Autodesk Inventor part; units mm, degrees
ref_plane "YZ Plane" through (0, 0, 0) normal (1, 0, 0) x (0, 1, 0)
ref_plane "XZ Plane" through (0, 0, 0) normal (0, 1, 0) x (-1, 0, 0)
ref_plane "XY Plane" through (0, 0, 0) normal (0, 0, 1) x (1, 0, 0)
sketch "Sketch1" plane through (0, 0, 0) normal (0, 1, 0) x (-1, 0, 0)
  circle A0 centre (0, 0) radius 175
  dimension "d0" = 350
extrude "Extrusion1" add sketch "Sketch1" along normal blind 10
sketch "Sketch2" plane through (0, 0, 0) normal (0, -1, 0) x (1, 0, 0)
  circle A0 centre (0, 0) radius 175
  circle A1 centre (0, 135) radius 25
  line L0 (-25, 135) -> (-25, 173.2051)
  line L1 (25, 135) -> (25, 173.2051)
  dimension "d3" = 50
  dimension "d4" = 135
extrude "Extrusion2" cut sketch "Sketch2" against normal through all contours L1 A1 L0 A0 | A1 picked at (-14.0746, 168.7936)
pattern_circular "Circular Pattern1" count 4 over 360 about axis through (0, 0, 0) along (0, 1, 0) of "Extrusion2"
properties part number "Base" material "Steel"
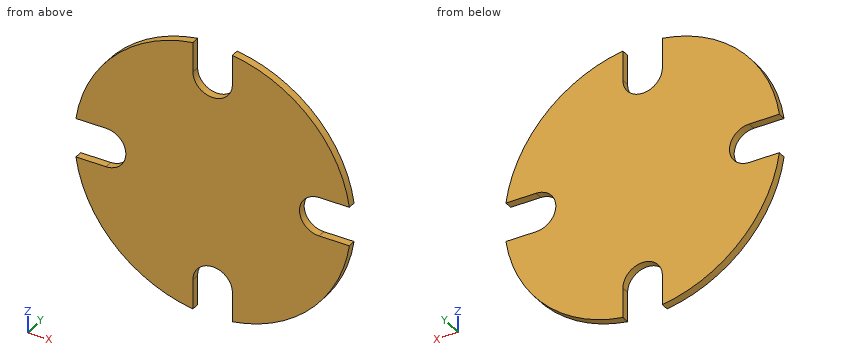
Check sheet for the modelled part. Datum: model origin and axes. Units: mm. Give positions to 0.01 mm unless a question says otherwise; leave off trailing zeros. Write each loop counter-clockwise with the first axis right and the second up, starting at its lowest first coordinate (ties: lowest second). Pieces come first, ordered by that corner, then holes.
Item 1: Gauge pin test, flat ends, axial feed: pin 1 (1.5 mm diameter, centred on y = 8, z = -119, fed in from +X); pin 2 (5 mm diameter, centred on y = 6, z = -151.5, fed in from +X); pin 3 (5 mm diameter, centred on x = 158.5, y = 5.5, fed in from +Z). Record the tip position at first contact, or that the pin passes through.
Item 2: Scan lines: L1, parallel to Z at x = 129.5, y = 5; L2, parallel to X at y = 4.25, z = -147; L3, parallel to Z at x = -117, y = 4.25. Record each from-to range of solid material in increasing order.
Item 3: Cross-section at D-D (z = 0). Enter the section's corners in (x, y), and give its area (3 significant figures).
Item 4: Cross-section at A-A (y = 2.5). Enter the section's corners in (x, z).
Item 5: Cross-section at C-C (x = 0). Enter the section's corners in (y, z), and give its area (3 significant figures).
Item 6: Cross-section at B-B (x = 152). Enter the section's corners in (y, z), and give its area (3 significant figures).
Report:
1. pin 1: stops at x = 129
1. pin 2: stops at x = 91.78
1. pin 3: stops at z = 79.3
2. L1: z = -117.71 to -24.39, 24.39 to 117.71
2. L2: x = -94.95 to -25, 25 to 94.95
2. L3: z = -130.14 to -17.35, 17.35 to 130.14
3. outline: (-110, 0) - (110, 0) - (110, 10) - (-110, 10) - close
3. area: 2,200 mm2
4. outline: (-173.21, -25) arc R175 ccw to (-25, -173.21) - (-25, -135) arc R25 cw to (25, -135) - (25, -173.21) arc R175 ccw to (173.21, -25) - (135, -25) arc R25 cw to (135, 25) - (173.21, 25) arc R175 ccw to (25, 173.21) - (25, 135) arc R25 cw to (-25, 135) - (-25, 173.21) arc R175 ccw to (-173.21, 25) - (-135, 25) arc R25 cw to (-135, -25) - close
5. outline: (0, -110) - (10, -110) - (10, 110) - (0, 110) - close
5. area: 2,200 mm2
6. outline: (0, -86.72) - (10, -86.72) - (10, -25) - (0, -25) - close; (0, 25) - (10, 25) - (10, 86.72) - (0, 86.72) - close
6. area: 1,230 mm2
